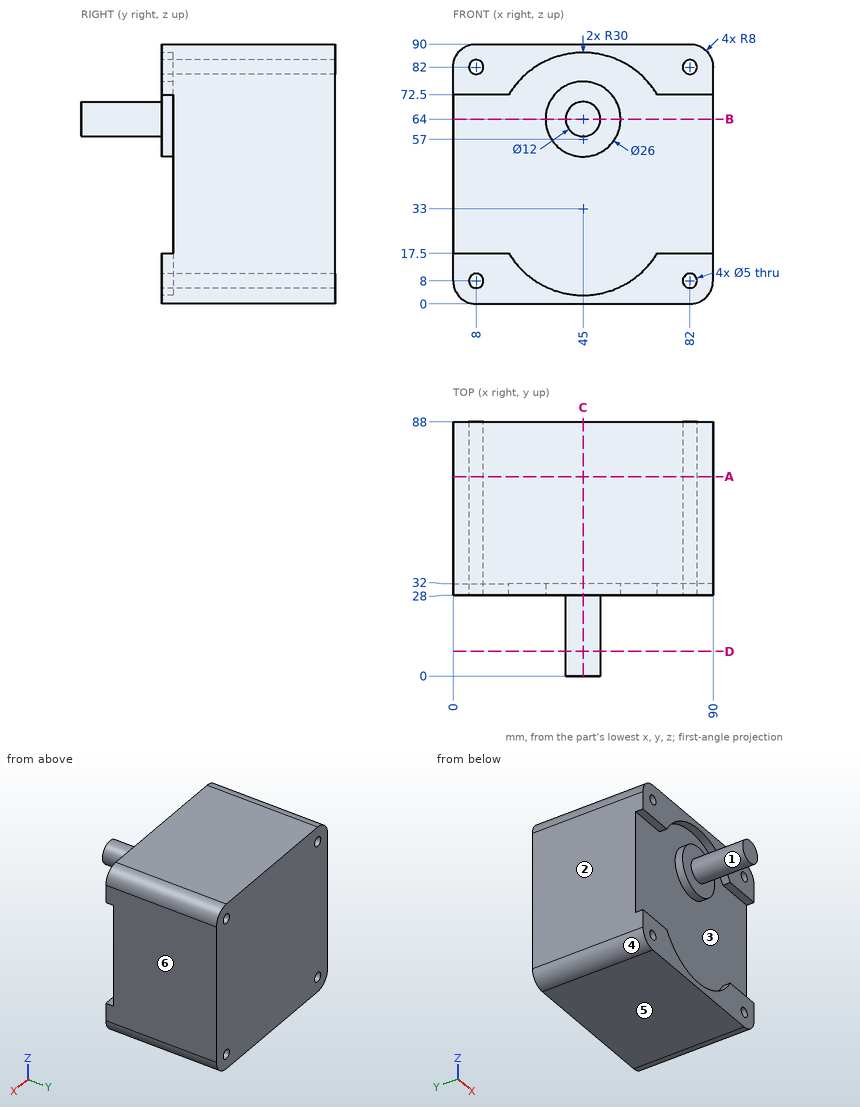
Check sheet for the drawn part. Datum: minimum x, y, z corner. Units: mm. A direction names the side the tool comes from. Round coordinates to 2 decimals unless told otherwise and drop trailing zeros. Write each loop counter-clockwise with the first axis right and the second up, starting at its lowest first coordinate (ties: lowest second). Pieces come first, ordered by that corner, then holes. Notation, with made-up numbers: (84, -21.75) -> (105, -21.75) arc R26 ccw to (105, 3.25) -> close; hole circle Ø3 at (64, 0). An arc over 180 degrees is marked (long way). One line per item, written item: value. Start each with the question number.
(1) Access from +Z, -Z, +X, -X, +Y, -Y to the whole of each face (thin tool, end or side, straight path). Record for the marked faces 1 and 2.
(2) Cross-section at D-D, the plane y = 8.5. Record the cut outline in (x, z), and give its area (3 significant figures).
(3) Cross-section at B-B, the plane z = 64. Record the cut outline in (x, y).
(4) Cross-section at A-A, the plane y = 69. Record the cut outline in (x, z).
(5) Go/stop test with flat-tipped pins: pin 1 Ø10 at (x, z) = (11, 29) entering from -Y; pin 2 Ø6.5 at (x, z) = (82, 82) entering from -Y; pin 3 Ø3 at (x, y) = (85, 30) entering from +Z. Record where each tip stops, or that it passes through.
(6) Scan lines: line 1 (Z direction, x = 8, y = 70); line 2 (Z direction, x = 80.5, y = 45.5); line 3 (Y direction, x = 4, z = 28). Record each from-to range of solid material in increasing order. Write a range as [from, to].
(7) Cross-section at C-C, the plane x = 45. Record the cut outline in (y, z), and give its area (3 significant figures).
(8) Draft check along X on the marked faces 3, 4, 5 and 6. Enter one of: +X half, -X half, draft (parallel to the pull), parting line (faces both ways), or undercut.
Answer:
1. face 1: -Y
1. face 2: +Z, -Z, -X, +Y, -Y
2. outline: circle Ø12 at (45, 64)
2. area: 113 mm²
3. outline: (0, 32) -> (32, 32) -> (32, 28) -> (39, 28) -> (39, 0) -> (51, 0) -> (51, 28) -> (58, 28) -> (58, 32) -> (90, 32) -> (90, 88) -> (0, 88) -> close
4. outline: (0, 8) arc R8 ccw to (8, 0) -> (82, 0) arc R8 ccw to (90, 8) -> (90, 82) arc R8 ccw to (82, 90) -> (8, 90) arc R8 ccw to (0, 82) -> close; hole circle Ø5 at (8, 8); hole circle Ø5 at (8, 82); hole circle Ø5 at (82, 8); hole circle Ø5 at (82, 82)
5. pin 1: y = 32
5. pin 2: y = 28
5. pin 3: z = 89.86
6. line 1: [0, 5.5], [10.5, 79.5], [84.5, 90]
6. line 2: [0, 6], [10, 80], [84, 90]
6. line 3: [32, 88]
7. outline: (0, 58) -> (28, 58) -> (28, 51) -> (32, 51) -> (32, 3) -> (28, 3) -> (28, 0) -> (88, 0) -> (88, 90) -> (28, 90) -> (28, 87) -> (32, 87) -> (32, 77) -> (28, 77) -> (28, 70) -> (0, 70) -> close
7. area: 5,500 mm²
8. face 3: undercut
8. face 4: -X half
8. face 5: draft
8. face 6: +X half
